```python
from build123d import *

# Parameters (mm, degrees)
F1_DEPTH  = 12.7
F2_W      = 19.4173352793
F2_H      = 11.3267796114
F3_DEPTH  = 5.08
F4_W      = 12.7
F4_H      = 4.7013934236
F5_DEPTH  = 7.62
F6_DEPTH  = 5.08
F7_W      = 17.6784014329
F7_H      = 9.7536002286
F8_DEPTH  = 5.08
F9_W      = 16.7640009895
F9_H      = 8.8392002508
F10_DEPTH = 5.08


with BuildPart() as f1:
    # F0 (on Front) → F1 (new body)
    with BuildSketch(Plane.XZ):
        Polygon((11.9880298153, 7.1389395744), (-11.7186363786, 7.1389395744), (-11.7186363786, -8.2165151834), (11.9880298153, -8.2165151834), (11.9880298153, -2.5592423044), align=None)
    extrude(amount=F1_DEPTH)

    # F2 (on face) → F3 (cut)
    with BuildSketch(Plane(origin=(0, 0, 0), x_dir=(-1, 0, 0), z_dir=(0, 1, 0))):
        with Locations((-0.2076723613, -0.6256373599)):
            Rectangle(F2_W, F2_H)
    extrude(amount=-F3_DEPTH, mode=Mode.SUBTRACT)

    # F4 (on face) → F5 (join)
    with BuildSketch(Plane(origin=(-11.7186363786, 0, 0), x_dir=(0, -1, 0), z_dir=(-1, 0, 0))):
        with Locations((6.35, -5.8658184716)):
            Rectangle(F4_W, F4_H)
    extrude(amount=F5_DEPTH)

    # F6 (add): a face of the model
    f6_faces = [f1.faces().sort_by_distance(p)[0] for p in [
        (0.2076723613, -5.08, -0.6256373599),
    ]]
    extrude(f6_faces, amount=F6_DEPTH)

    # F7 (on face) → F8 (cut)
    with BuildSketch(Plane.XZ.offset(12.7)):
        with Locations((-0.1524002291, -0.6095997524)):
            Rectangle(F7_W, F7_H)
    extrude(amount=-F8_DEPTH, mode=Mode.SUBTRACT)

    # F9 (on face) → F10 (cut)
    with BuildSketch(Plane(origin=(0, 0, 0), x_dir=(-1, 0, 0), z_dir=(0, 1, 0))):
        with Locations((-4.657e-07, -0.7620002143)):
            Rectangle(F9_W, F9_H)
    extrude(amount=-F10_DEPTH, mode=Mode.SUBTRACT)


solid = f1.part
```
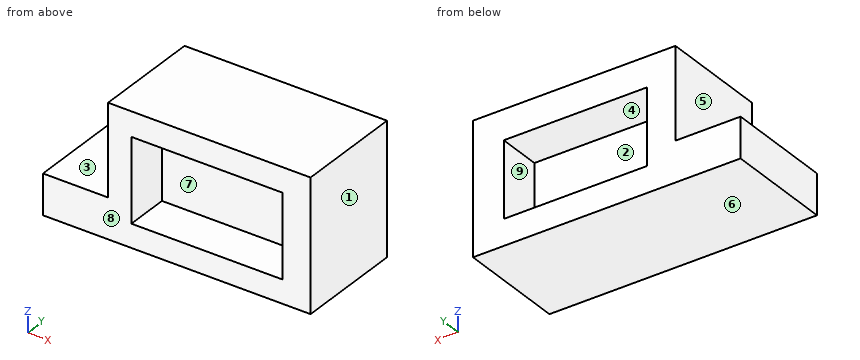
Geometry: final body of the model. Coordinates: model frame, mm. Face numbers are marked on the shaded views. A direction names the side the tool comes from. Round coordinates to 2 decimals unless told otherwise and drop trailing zeros. Write each loop counter-clockwise with the first axis right and the second up, starting at its lowest first coordinate (ties: lowest second). Pieces come first, ordered by that corner, then holes.
Item 1: Set-up query: the marked faces 5, 6, 7, 8 and 9. Return all of +Z, -Z, +X, -X, +Y, -Y with unobstructed straight access to the full face (end or side cutting, diameter ignored); none if empty.
Item 2: Section query C-C (x = 4). Return loops of the section in (y, z).
Item 3: Section query B-B (z = 0). Return loops of the section in (x, y).
Item 4: Mould query, pull axis X, two halves, no side actions, for the marked faces 1, 2, 3 and 4. Classes: +X half, -X half, draft (parallel to the pull), parting line (faces both ways), or undercut.
Item 5: Section query A-A (y = -4.25). Return loops of the section in (x, z), plus the area to 3 significant figures.
Item 6: Material intervals for L1, parallel to X at y = -10.25, z = -4.25; L2, parallel to X at y = -8.5, z = -2.5; L3, parallel to Z at x = -3.5, y = -11, sorted ascending.
Item 7: Pin query (flat end, axial travel): P1, Ø2.5, axis at y = -3.5, z = 0, coming from the -X side; P2, Ø2.5, axis at x = -13.5, y = -4.5, coming from the +Z side; P3, Ø4, axis at x = -4.5, z = -3, coming from the -Y side. Return the tip coordinate at first contact, or that it passes through.
Item 8: Section query D-D (y = -6.25). Return loops of the section in (x, z), plus the area to 3 significant figures.
Completed:
1. face 5: +Z, -X, +Y, -Y
1. face 6: -Z, +X, -X, +Y, -Y
1. face 7: -Y
1. face 8: +Z, -Z, +X, -X, -Y
1. face 9: +Y
2. outline: (-12.7, -8.22) - (0, -8.22) - (0, -5.18) - (-5.08, -5.18) - (-5.08, 3.66) - (0, 3.66) - (0, 7.14) - (-12.7, 7.14) - (-12.7, 4.27) - (-7.62, 4.27) - (-7.62, -5.49) - (-12.7, -5.49) - close
3. outline: (-11.72, -12.7) - (-8.99, -12.7) - (-8.99, -7.62) - (8.69, -7.62) - (8.69, -12.7) - (11.99, -12.7) - (11.99, 0) - (8.38, 0) - (8.38, -5.08) - (-8.38, -5.08) - (-8.38, 0) - (-11.72, 0) - close
4. face 1: +X half
4. face 2: undercut
4. face 3: draft
4. face 4: undercut
5. outline: (-19.34, -8.22) - (11.99, -8.22) - (11.99, 7.14) - (-11.72, 7.14) - (-11.72, -3.52) - (-19.34, -3.52) - close; hole (-8.38, -5.18) - (8.38, -5.18) - (8.38, 3.66) - (-8.38, 3.66) - close
5. area: 252 mm2
6. L1: x = -19.34 to -8.99, 8.69 to 11.99
6. L2: x = -11.72 to -8.99, 8.69 to 11.99
6. L3: z = -8.22 to -5.49, 4.27 to 7.14
7. P1: stops at x = -11.72
7. P2: stops at z = -3.52
7. P3: stops at y = -7.62
8. outline: (-19.34, -8.22) - (11.99, -8.22) - (11.99, 7.14) - (-11.72, 7.14) - (-11.72, -3.52) - (-19.34, -3.52) - close
8. area: 400 mm2
